Autodesk Inventor part; units mm, degrees
ref_plane "YZ Plane" through (0, 0, 0) normal (1, 0, 0) x (0, 1, 0)
ref_plane "XZ Plane" through (0, 0, 0) normal (0, 1, 0) x (-1, 0, 0)
ref_plane "XY Plane" through (0, 0, 0) normal (0, 0, 1) x (1, 0, 0)
sketch "Sketch4" plane through (0, 0, 0) normal (0, 1, 0) x (-1, 0, 0)
  line L0 (72.5, -25) -> (-72.5, -25)
  line L1 (-72.5, -25) -> (-72.5, 25)
  line L2 (-72.5, 25) -> (72.5, 25)
  line L3 (72.5, 25) -> (72.5, -25)
  line L4 (72.5, -25) -> (-72.5, 25) construction
  line L5 (-72.5, -25) -> (72.5, 25) construction
  line L6 (102.5, -40) -> (-102.5, -40)
  line L7 (-102.5, -40) -> (-102.5, 40)
  line L8 (-102.5, 40) -> (102.5, 40)
  line L9 (102.5, 40) -> (102.5, -40)
  line L10 (102.5, -40) -> (-102.5, 40) construction
  line L11 (-102.5, -40) -> (102.5, 40) construction
  circle A0 centre (82.5, 0) radius 5
  circle A1 centre (-82.5, 0) radius 5
  line L12 (0, -25) -> (0, 25) construction
  point P0 (0, 0)
  dimension "d23" = 145
  dimension "d24" = 50
  dimension "d25" = 205
  dimension "d26" = 80
  dimension "d27" = 165
  dimension "d28" = 10
extrude "Extrusion3" add sketch "Sketch4" along normal blind 10
fillet "Fillet2" radius 6 4 edges at (-72.5, 5, -25) (72.5, 5, -25) (72.5, 5, 25) (-72.5, 5, 25)
properties part number "DMF 01 54 lower sheet v2.1"
Check sheet for the modelled part. Datum: model origin and axes. Units: mm. A direction names the side the tool comes from. Round coordinates to 2 decimals unless told otherwise and drop trailing zeros. Write each loop counter-clockwise with the first axis right and the second up, starting at its lowest first coordinate (ties: lowest second). Pieces come first, ordered by that corner, then holes. Notation, with made-up numbers: (12.25, -18.5) -> (56.25, -18.5) arc R12 cw to (56.25, -5.5) -> close; hole circle Ø1 at (26.5, 89). An arc over 180 degrees is marked (long way). One line per question, with ' | ' between items. Start each with the question number.
1. Release check for a two-part mould opening along X. For faces 3 (the face through (1, 5, 40)), 4 (the face through (-102.5, 5, 1)), 5 (the face through (-87.119, 4.93, 1.915)) record: +X half, -X half, draft (parallel to the pull), parting line (faces both ways), or undercut.
2. Sectioned sample at C-C, the plane y = 3.25. Record the cut outline in (x, z).
3. Sectioned sample at A-A, the plane x = 4. Record the cut outline in (y, z).
4. Set-up check for faces 1 (the face through (-1, 5, -25)), 2 (the face through (1, 0, 27)): record each of +Z, -Z, +X, -X, +Y, -Y from which the full face is reachable in a straight line by a thin tool's end or side.
5. Sectioned sample at B-B, the plane z = 0. Record the cut outline in (x, y).
6. Sectioned sample at D-D, the plane z = 14. Record the cut outline in (x, y).
7. Scan lines: line 1 along Z through (x, y) = (21, 2.25); line 2 along X through (y, z) = (5.5, 8.5); line 3 along Z through (x, y) = (82.5, 2). Record each from-to range of solid material in increasing order. Write a range as from..to.
Taken from the geometry:
1) face 3: draft | face 4: -X half | face 5: undercut
2) outline: (-102.5, -40) -> (102.5, -40) -> (102.5, 40) -> (-102.5, 40) -> close; hole circle Ø10 at (-82.5, 0); hole (-72.5, -19) arc R6 ccw to (-66.5, -25) -> (66.5, -25) arc R6 ccw to (72.5, -19) -> (72.5, 19) arc R6 ccw to (66.5, 25) -> (-66.5, 25) arc R6 ccw to (-72.5, 19) -> close; hole circle Ø10 at (82.5, 0)
3) outline: (0, -40) -> (10, -40) -> (10, -25) -> (0, -25) -> close; (0, 25) -> (10, 25) -> (10, 40) -> (0, 40) -> close
4) face 1: +Y, -Y | face 2: +Z, -Z, +X, -X, -Y
5) outline: (-102.5, 0) -> (-87.5, 0) -> (-87.5, 10) -> (-102.5, 10) -> close; (-77.5, 0) -> (-72.5, 0) -> (-72.5, 10) -> (-77.5, 10) -> close; (72.5, 0) -> (77.5, 0) -> (77.5, 10) -> (72.5, 10) -> close; (87.5, 0) -> (102.5, 0) -> (102.5, 10) -> (87.5, 10) -> close
6) outline: (-102.5, 0) -> (-72.5, 0) -> (-72.5, 10) -> (-102.5, 10) -> close; (72.5, 0) -> (102.5, 0) -> (102.5, 10) -> (72.5, 10) -> close
7) line 1: z = -40..-25, 25..40 | line 2: x = -102.5..-72.5, 72.5..102.5 | line 3: z = -40..-5, 5..40
